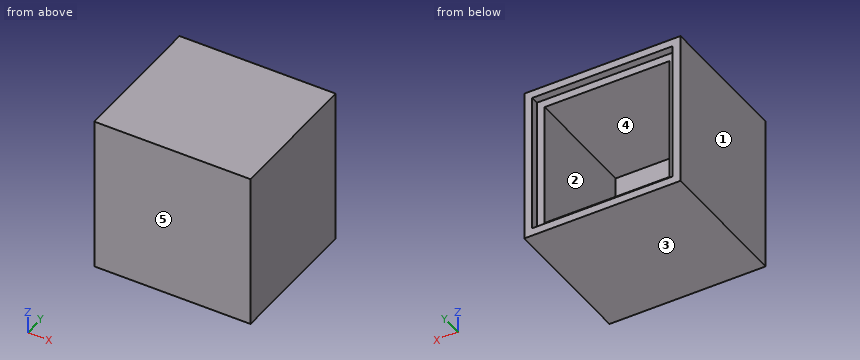
from build123d import *

# Parameters (mm, degrees)
CROQUIS1_W              = 50
CROQUIS1_H              = 50
SALIENTE_EXTRUIR1_DEPTH = 45
CROQUIS2_W              = 40
CROQUIS2_H              = 40
CORTAR_EXTRUIR1_DEPTH   = 40
CROQUIS3_W              = 45
CROQUIS3_H              = 45
CORTAR_EXTRUIR2_DEPTH   = 2.5


with BuildPart() as part:
    # Croquis1 → Saliente-Extruir1 (new body)
    with BuildSketch(Plane(origin=(0, 0, 0), x_dir=(1, 0, 0), z_dir=(0, 1, 0))):
        Rectangle(CROQUIS1_W, CROQUIS1_H)
    extrude(amount=SALIENTE_EXTRUIR1_DEPTH)

    # Croquis2 → Cortar-Extruir1 (cut)
    with BuildSketch(Plane(origin=(0, 45, 0), x_dir=(1, 0, 0), z_dir=(0, 1, 0))):
        Rectangle(CROQUIS2_W, CROQUIS2_H)
    extrude(amount=-CORTAR_EXTRUIR1_DEPTH, mode=Mode.SUBTRACT)

    # Croquis3 → Cortar-Extruir2 (cut)
    with BuildSketch(Plane(origin=(0, 45, 0), x_dir=(1, 0, 0), z_dir=(0, 1, 0))):
        Rectangle(CROQUIS3_W, CROQUIS3_H)
    extrude(amount=-CORTAR_EXTRUIR2_DEPTH, mode=Mode.SUBTRACT)


solid = part.part
The listing builds one solid part. Answer for the finished solid, in the listing's coordinates (mm). Face numbers are marked on the shaded views. A direction names the side the tool comes from. Round coordinates to 2 decimals unless told otherwise and drop trailing zeros. Write each loop counter-clockwise with the first axis right and the second up, starting at its lowest first coordinate (ties: lowest second). Pieces come first, ordered by that corner, then holes. Notation, with made-up numbers: (76, -6.75) - (97, -6.75) arc R15 ccw to (97, 16.25) - close; hole circle Ø6 at (23.5, 5.5). An arc over 180 degrees is marked (long way). Use a Markdown table: item, result. Add a question column.
1. Consider line 1 (X direction, y = 25.5, z = 13.5); line 2 (Y direction, x = 14.5, z = 11.5). Determine where each line is inside the solid, lowest interval first.
2. A tool of negligible diameter and unlimited length cuts with its end or side. For the marked faces 4 and 5, from which of +Z, -Z, +X, -X, +Y, -Y can it reach the whole face along a straight path? Write none if from no direction.
3. The part is cut by section D-D (x = -21). Write down the section's boundary in (y, z), and give its area (3 significant figures).
4. The part is cut by section B-B (x = 18.5). Write down the section's boundary in (y, z).
5. For a pull along X with two mould halves and no side action, classify the marked faces 1, 2 and 3 as +X half, -X half, draft (parallel to the pull), parting line (faces both ways), or undercut.
6. The part is cut by section A-A (y = 36). Write down the section's boundary in (x, z), and give its area (3 significant figures).
7. The part is cut by section C-C (z = -18.5). Write down the section's boundary in (x, y), and give its area (4 significant figures).
8. Flat-ended cylindrical pins translate along their axes: P1, Ø20, axis at x = 8, z = -3, coming from the +Y side; P2, Ø22.5, axis at x = -9.5, z = 10.5, coming from the +Y side; P3, Ø1, axis at x = -11.5, z = -18, coming from the -Y side. Find the tip coordinate at first contact, or state that the pin passes through.
Reported:
| question | item | result |
|---|---|---|
| 1 | line 1 | -25 to -20, 20 to 25 |
| 1 | line 2 | 0 to 5 |
| 2 | face 4 | +Y |
| 2 | face 5 | +Z, -Z, +X, -X, -Y |
| 3 | outline | (0, -25) - (45, -25) - (45, -22.5) - (42.5, -22.5) - (42.5, 22.5) - (45, 22.5) - (45, 25) - (0, 25) - close |
| 3 | area | 2,140 mm^2 |
| 4 | outline | (0, -25) - (45, -25) - (45, -22.5) - (42.5, -22.5) - (42.5, -20) - (5, -20) - (5, 20) - (42.5, 20) - (42.5, 22.5) - (45, 22.5) - (45, 25) - (0, 25) - close |
| 5 | face 1 | -X half |
| 5 | face 2 | undercut |
| 5 | face 3 | draft |
| 6 | outline | (-25, -25) - (25, -25) - (25, 25) - (-25, 25) - close; hole (-20, -20) - (20, -20) - (20, 20) - (-20, 20) - close |
| 6 | area | 900 mm^2 |
| 7 | outline | (-25, 0) - (25, 0) - (25, 45) - (22.5, 45) - (22.5, 42.5) - (20, 42.5) - (20, 5) - (-20, 5) - (-20, 42.5) - (-22.5, 42.5) - (-22.5, 45) - (-25, 45) - close |
| 7 | area | 637.5 mm^2 |
| 8 | P1 | y = 5 |
| 8 | P2 | y = 42.5 |
| 8 | P3 | y = 0 |
